Verification items for the finished model (mm, model axes). Coordinates: 2 decimals unless noted, no trailing zeros. Loops run counter-clockwise (first coordinate to the right, second up) from the corner with the lowest first, then second, coordinate; pieces in that order, holes last. Notation, with made-up numbers: (-12, -35.5) -> (45, -35.5) arc R25 cw to (45, -2.5) -> close; hole circle Ø8 at (39.5, 16.5). An arc over 180 degrees is marked (long way). Answer as a JSON object with one key per item and string values. Group by question number.
Q1. Cross-section at D-D on z = 2. Record the boundary of the cut face in (x, y).
Q2. Cross-section at B-B on x = 0. Record the boundary of the cut face in (y, z).
Q3. Cross-section at A-A on z = 20. Record the boundary of the cut face in (x, y).
Q4. Release check for a two-part mould opening along Z. For faces 1 (the flat face through (0, 0, 40)), 2 (the flat face through (0, 0, -40)), 3 (the cylindrical face through (1.18, 0.09, -36.29)) record: released by +Z, released by -Z, zero draft, split by the parting line, or undercut.
Q5. Gauge pin test, flat end, axial feed: pin 1 Ø2 at (x, z) = (0, -20) entering from -Y. Record the tip position at first contact, or that the pin passes through.
Q6. Cross-section at C-C on x = -5. Record the boundary of the cut face in (y, z).
Q7. Scan lines: L1, parallel to X at y = 3.5, z = -35; L2, parallel to Z at x = 6, y = 3.5; L3, parallel to X at y = -1.75, z = -19. Record each from-to range of solid material in increasing order.
```python
from build123d import *

# Parameters (mm, degrees)
SKETCH_1_W               = 13
SKETCH_1_H               = 80
EXTRUDE_1_DEPTH          = 6.5
CUT_EXTRUDE_1_DEPTH      = 42.042660732
CUT_EXTRUDE_1_DEPTH_BACK = 42.042660732
SKETCH_4_R               = 1.75
CUT_EXTRUDE_2_DEPTH      = 42.042660732


with BuildPart() as part:
    # 스케치1 → 보스-돌출1 (new, symmetric)
    with BuildSketch(Plane(origin=(0, 0, 0), x_dir=(1, 0, 0), z_dir=(0, 1, 0))):
        Rectangle(SKETCH_1_W, SKETCH_1_H)
    extrude(amount=EXTRUDE_1_DEPTH, both=True)

    # 스케치3 → 컷-돌출1 (cut, two sides: drawn at the far end of the back side and taken through both)
    with BuildSketch(Plane(origin=(0, 0, 0), x_dir=(0, 0, -1), z_dir=(1, 0, 0)).offset(-CUT_EXTRUDE_1_DEPTH_BACK)):
        with BuildLine():
            ThreePointArc((0, 2.41091269), (0.55817077, 1.262438117), (0.75, 0))
            Line((0.75, 0), (7.75, 0))
            ThreePointArc((7.75, 0), (4.762438117, 4.05817077), (0, 2.41091269))
        make_face()
        with BuildLine():
            ThreePointArc((0, -2.41091269), (0.55817077, -1.262438117), (0.75, 0))
            Line((0.75, 0), (-0.75, 0))
            ThreePointArc((-0.75, 0), (-0.55817077, -1.262438117), (0, -2.41091269))
        make_face()
        with BuildLine():
            Line((-0.75, 0), (0.75, 0))
            ThreePointArc((0.75, 0), (0.55817077, 1.262438117), (0, 2.41091269))
            ThreePointArc((0, 2.41091269), (-0.55817077, 1.262438117), (-0.75, 0))
        make_face()
        with BuildLine():
            Line((7.75, 0), (0.75, 0))
            ThreePointArc((0.75, 0), (0.55817077, -1.262438117), (0, -2.41091269))
            ThreePointArc((0, -2.41091269), (4.762438117, -4.05817077), (7.75, 0))
        make_face()
        with BuildLine():
            ThreePointArc((0, -2.41091269), (-0.55817077, -1.262438117), (-0.75, 0))
            Line((-0.75, 0), (-7.75, 0))
            ThreePointArc((-7.75, 0), (-4.762438117, -4.05817077), (0, -2.41091269))
        make_face()
        with BuildLine():
            Line((-7.75, 0), (-0.75, 0))
            ThreePointArc((-0.75, 0), (-0.55817077, 1.262438117), (0, 2.41091269))
            ThreePointArc((0, 2.41091269), (-4.762438117, 4.05817077), (-7.75, 0))
        make_face()
    extrude(amount=CUT_EXTRUDE_1_DEPTH + CUT_EXTRUDE_1_DEPTH_BACK, mode=Mode.SUBTRACT)

    # 스케치4 → 컷-돌출2 (cut, symmetric)
    with BuildSketch(Plane(origin=(0, 0, 0), x_dir=(1, 0, 0), z_dir=(0, 1, 0))):
        with Locations(Location((0, 35, 0), (0, 0, 270))):
            Circle(SKETCH_4_R)
        with Locations(Location((0, 20, 0), (0, 0, 270))):
            Circle(SKETCH_4_R)
    cut_extrude_2 = extrude(amount=CUT_EXTRUDE_2_DEPTH, both=True, mode=Mode.SUBTRACT)

    # 대칭 복사1: 컷-돌출2 across plane
    add(cut_extrude_2.mirror(Plane.XY), mode=Mode.SUBTRACT)


solid = part.part
```
Computed values:
{
 "1": {"outline": "(-6.5, -6.5) -> (6.5, -6.5) -> (6.5, -3.98) -> (-6.5, -3.98) -> close; (-6.5, 3.98) -> (6.5, 3.98) -> (6.5, 6.5) -> (-6.5, 6.5) -> close"},
 "2": {"outline": "(-6.5, -40) -> (6.5, -40) -> (6.5, -36.75) -> (-6.5, -36.75) -> close; (-6.5, -33.25) -> (6.5, -33.25) -> (6.5, -21.75) -> (-6.5, -21.75) -> close; (-6.5, -18.25) -> (6.5, -18.25) -> (6.5, 18.25) -> (-6.5, 18.25) -> close; (-6.5, 21.75) -> (6.5, 21.75) -> (6.5, 33.25) -> (-6.5, 33.25) -> close; (-6.5, 36.75) -> (6.5, 36.75) -> (6.5, 40) -> (-6.5, 40) -> close; hole (-2.41, 0) arc R4.25 ccw (long way) to (2.41, 0) arc R4.25 ccw (long way) to start"},
 "3": {"outline": "(-6.5, -6.5) -> (-1.75, -6.5) -> (-1.75, 6.5) -> (-6.5, 6.5) -> close; (1.75, -6.5) -> (6.5, -6.5) -> (6.5, 6.5) -> (1.75, 6.5) -> close"},
 "4": {"face 1": "released by +Z", "face 2": "released by -Z", "face 3": "undercut"},
 "5": {"pin 1": "passes through"},
 "6": {"outline": "(-6.5, -40) -> (6.5, -40) -> (6.5, 40) -> (-6.5, 40) -> close; hole (-2.41, 0) arc R4.25 ccw (long way) to (2.41, 0) arc R4.25 ccw (long way) to start"},
 "7": {"L1": "x = -6.5 to -1.75, 1.75 to 6.5", "L2": "z = -40 to -5.91, -1.09 to 1.09, 5.91 to 40", "L3": "x = -6.5 to -1.44, 1.44 to 6.5"}
}
